The model under review builds one solid part; all positions refer to its coordinate system, in mm. Face numbers are marked on the shaded views. A direction names the side the tool comes from. Round coordinates to 2 decimals unless told otherwise and drop trailing zeros. Loops run counter-clockwise (first coordinate to the right, second up) from the corner with the lowest first, then second, coordinate; pieces in that order, holes last. Notation, with made-up numbers: (4.25, 75.25) -> (16.25, 75.25) arc R22 cw to (16.25, 101.25) -> close; hole circle Ø8 at (45, -25.75). An arc over 180 degrees is marked (long way). Return JSON: item names as keys, results as strings. Group by question number.
```python
from build123d import *

# Parameters (mm, degrees)
SKETCH1_W           = 47.35
SKETCH1_H           = 10.675
BOSS_EXTRUDE1_DEPTH = 3.175
SKETCH2_W           = 8.675
SKETCH2_H           = 3.175
SKETCH2_W_2         = 10
SKETCH2_H_2         = 1.5875
CUT_EXTRUDE1_DEPTH  = 4.175


with BuildPart() as part:
    # Sketch1 → Boss-Extrude1 (new body)
    with BuildSketch(Plane(origin=(0, 0, 0), x_dir=(1, 0, 0), z_dir=(0, 1, 0))):
        with Locations((23.675, 5.3375)):
            Rectangle(SKETCH1_W, SKETCH1_H)
    extrude(amount=BOSS_EXTRUDE1_DEPTH)

    # Sketch2 → Cut-Extrude1 (cut, through all)
    with BuildSketch(Plane.XZ):
        with Locations((43.0125, -1.5875)):
            Rectangle(SKETCH2_W, SKETCH2_H)
        with Locations((23.675, -1.5875)):
            Rectangle(SKETCH2_W_2, SKETCH2_H)
        with Locations((4.3375, -1.5875)):
            Rectangle(SKETCH2_W, SKETCH2_H)
        with Locations((43.0125, -9.88125)):
            Rectangle(SKETCH2_W, SKETCH2_H_2)
        with Locations((23.675, -9.88125)):
            Rectangle(SKETCH2_W_2, SKETCH2_H_2)
        with Locations((4.3375, -9.88125)):
            Rectangle(SKETCH2_W, SKETCH2_H_2)
    extrude(amount=-CUT_EXTRUDE1_DEPTH, mode=Mode.SUBTRACT)


solid = part.part
```
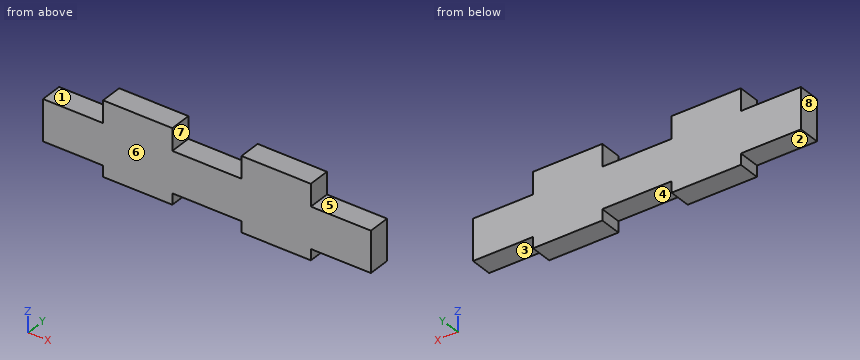
1. Draft analysis for pull direction X (two halves, no side actions). For the marked faces 6, 7 and 8, state which applies: pulls with the +X half, pulls with the -X half, needs draft (parallel to the pull), parting line crosses it, or undercut.
2. We need section B-B, the plane x = 20. Write out the cut boundary in (y, z) (1 decimal), then the cut area to 3 significant figures.
3. Tool access review of the marked faces 1, 2, 3, 4 and 5: name each direction out of +Z, -Z, +X, -X, +Y, -Y from which nothing blocks a thin tool from reaching the whole face with its end or side.
4. For P1, Ø1, axis at y = 1, z = -1, coming from the -X side (3 decimals); P2, Ø0.5, axis at y = 1.5, z = -10, coming from the +X side (3 decimals); P3, Ø1.6, axis at x = 24, y = 1.5, coming from the +Z side (3 decimals), all flat-tipped, find the tip position at first contact; note any pin that passes through.
5. Wall thickness on line 1 (X direction, y = 0.9, z = -2) (3 decimals); line 2 (Z direction, x = 21, y = 0.4) (1 decimal): over which ranges is each line inside the solid? List them lowest first.
Check sheet entries:
{
 "1": {"face 6": "needs draft", "face 7": "undercut", "face 8": "pulls with the -X half"},
 "2": {"outline": "(0, -9.1) -> (3.2, -9.1) -> (3.2, -3.2) -> (0, -3.2) -> close", "area": "18.8 mm²"},
 "3": {"face 1": "+Z, -X, +Y, -Y", "face 2": "-Z, -X, +Y, -Y", "face 3": "-Z, +X, +Y, -Y", "face 4": "-Z, +Y, -Y", "face 5": "+Z, +X, +Y, -Y"},
 "4": {"P1": "stops at x = 8.675", "P2": "stops at x = 38.675", "P3": "stops at z = -3.175"},
 "5": {"line 1": "x = 8.675 to 18.675, 28.675 to 38.675", "line 2": "z = -9.1 to -3.2"}
}
